Geometry check sheet. Reference: the model listing, model coordinates, mm. Round coordinates to 2 decimals unless told otherwise and drop trailing zeros. Loops run counter-clockwise (first coordinate to the right, second up) from the corner with the lowest first, then second, coordinate; pieces in that order, holes last. Notation, with made-up numbers: (-8, 23.25) -> (18, 23.25) arc R13 cw to (18, 27.25) -> close; hole circle Ø11 at (56.25, 36). An arc over 180 degrees is marked (long way). Use a Markdown table: item, result. Add a question column.
Q1. Sectioned sample at B-B, the plane x = 148. Enter the section's corners in (y, z).
Q2. Gauge pin test, flat ends, axial feed: P1, Ø4, axis at x = 190.5, y = 12.7, coming from the -Z side; P2, Ø6.5, axis at x = 190.5, y = 38.1, coming from the -Z side; P3, Ø2, axis at x = 52, z = 5.5, coming from the +Y side; P4, Ø2, axis at y = 53.5, z = 5.5, coming from the -X side. Record the tip position at first contact, or that the pin passes through.
Q3. Sectioned sample at D-D, the plane y = 282. Enter the section's corners in (x, z), then the cut area to 3 significant figures.
Q4. Material ranges on L1, parallel to X at y = 106.5, z = 0.5; L2, parallel to Y at x = 112.5, z = 2.25; L3, parallel to X at y = 170.5, z = 5.25, recorded low to high.
Q5. Sectioned sample at A-A, the plane y = 73.5. Enter the section's corners in (x, z), then the cut area to 3 significant figures.
Q6. Sectioned sample at C-C, the plane z = 5. Give the number of separate pieces and of enclosed holes in the cut face, then the cut area to 3 significant figures.
```python
from build123d import *

# Parameters (mm, degrees)
BOSS_EXTRUDE1_DEPTH = 6.35
SKETCH2_R           = 2.4892
CUT_EXTRUDE1_DEPTH  = 7.35
SKETCH4_R           = 2.4892
BOSS_EXTRUDE2_DEPTH = 6.35
FILLET1_R           = 6.35


with BuildPart() as part:
    # Sketch1 → Boss-Extrude1 (new body)
    with BuildSketch(Plane.XY):
        Polygon((0, 25.4), (177.8, 304.8), (203.2, 304.8), (203.2, 0), (0, 0), align=None)
    extrude(amount=BOSS_EXTRUDE1_DEPTH)

    # Sketch2 → Cut-Extrude1 (cut, through all)
    with BuildSketch(Plane.XY.offset(6.35)):
        with Locations((190.5, 12.7)):
            Circle(SKETCH2_R)
        with Locations((165.1, 12.7)):
            Circle(SKETCH2_R)
        with Locations((139.7, 12.7)):
            Circle(SKETCH2_R)
        with Locations((114.3, 12.7)):
            Circle(SKETCH2_R)
        with Locations((88.9, 12.7)):
            Circle(SKETCH2_R)
        with Locations((63.5, 12.7)):
            Circle(SKETCH2_R)
        with Locations((38.1, 12.7)):
            Circle(SKETCH2_R)
        with Locations((190.5, 38.1)):
            Circle(SKETCH2_R)
        with Locations((190.5, 63.5)):
            Circle(SKETCH2_R)
        with Locations((190.5, 88.9)):
            Circle(SKETCH2_R)
        with Locations((190.5, 114.3)):
            Circle(SKETCH2_R)
        with Locations((190.5, 139.7)):
            Circle(SKETCH2_R)
        with Locations((190.5, 165.1)):
            Circle(SKETCH2_R)
        with Locations((190.5, 190.5)):
            Circle(SKETCH2_R)
        with Locations((190.5, 215.9)):
            Circle(SKETCH2_R)
        with Locations((190.5, 241.3)):
            Circle(SKETCH2_R)
        with Locations((190.5, 266.7)):
            Circle(SKETCH2_R)
        with Locations((190.5, 292.1)):
            Circle(SKETCH2_R)
        with Locations((12.7, 12.7)):
            Circle(SKETCH2_R)
        Polygon((22.580146513, 25.4), (177.8, 25.4), (177.8, 269.316912623), align=None)
    extrude(amount=-CUT_EXTRUDE1_DEPTH, mode=Mode.SUBTRACT)

    # Sketch4 → Boss-Extrude2 (add)
    with BuildSketch(Plane(origin=(0, 0, 0), x_dir=(-1, 0, 0), z_dir=(0, 0, -1))):
        Polygon((-107.95, 25.4), (-107.95, 159.552626909), (-127, 189.488341195), (-127, 25.4), align=None)
        with Locations((-117.475, 88.9)):
            Circle(SKETCH4_R, mode=Mode.SUBTRACT)
        with Locations((-117.475, 114.3)):
            Circle(SKETCH4_R, mode=Mode.SUBTRACT)
    extrude(amount=-BOSS_EXTRUDE2_DEPTH)

    # Fillet1
    fillet1_edges = [part.edges().sort_by_distance(p)[0] for p in [
        (127, 25.4, 3.175),
        (127, 189.488341195, 3.175),
        (107.95, 159.552626909, 3.175),
        (107.95, 25.4, 3.175),
        (22.580146513, 25.4, 3.175),
        (177.8, 269.316912623, 3.175),
        (177.8, 25.4, 3.175),
        (203.2, 0, 3.175),
        (0, 0, 3.175),
        (0, 25.4, 3.175),
        (177.8, 304.8, 3.175),
        (203.2, 304.8, 3.175),
    ]]
    fillet(fillet1_edges, radius=FILLET1_R)


solid = part.part
```
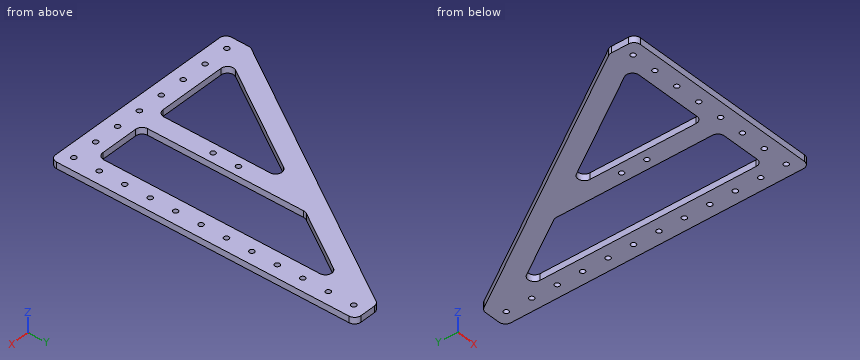
Values:
| question | item | result |
|---|---|---|
| 1 | outline | (0, 0) -> (25.4, 0) -> (25.4, 6.35) -> (0, 6.35) -> close; (222.49, 0) -> (257.97, 0) -> (257.97, 6.35) -> (222.49, 6.35) -> close |
| 2 | P1 | through |
| 2 | P2 | z = 0 |
| 2 | P3 | y = 108.69 |
| 2 | P4 | x = 17.25 |
| 3 | outline | (163.29, 0) -> (203.2, 0) -> (203.2, 6.35) -> (163.29, 6.35) -> close |
| 3 | area | 253 mm^2 |
| 4 | L1 | 51.61 to 74.19, 107.95 to 127, 177.8 to 203.2 |
| 4 | L2 | 0 to 10.98, 14.42 to 202.19 |
| 4 | L3 | 92.34 to 127, 177.8 to 203.2 |
| 5 | outline | (30.61, 0) -> (53.19, 0) -> (53.19, 6.35) -> (30.61, 6.35) -> close; (107.95, 0) -> (127, 0) -> (127, 6.35) -> (107.95, 6.35) -> close; (177.8, 0) -> (203.2, 0) -> (203.2, 6.35) -> (177.8, 6.35) -> close |
| 5 | area | 426 mm^2 |
| 6 | separate pieces | 1 |
| 6 | enclosed holes | 23 |
| 6 | area | 20,800 mm^2 |
